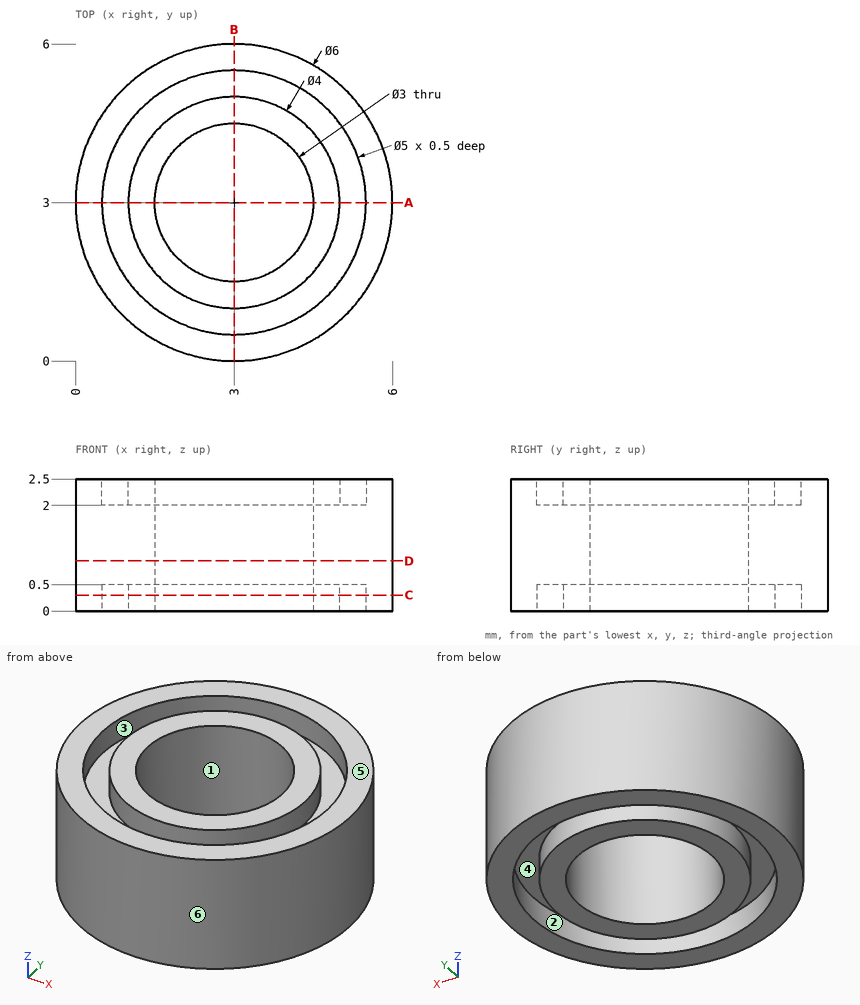
The figure shows three views and two pictorial views of one solid part (mm, origin at its lowest corner). Answer the questions. A direction names the side the tool comes from. Round coordinates to 2 decimals unless told otherwise and drop trailing zeros. Order: outer loops, then holes, each group sorted by start corner. A loop starts at its lowest first (then second) coordinate and runs counter-clockwise, first axis right, second up. Notation, with made-up numbers: M 33,40.25 L 61,40.25 A23 cw 61,61.25 Z; hole C -28.75,3 d1. An arc over 180 degrees is marked long. Answer in a Markdown table with one row per item. Add a question column.
1) The part is cut by section A-A on y = 3. Determine the outline of the cut face in (x, z), plus the area to 3 significant figures.
2) Which of the six approach directions +Z, -Z, +X, -X, +Y, -Y give full straight-line access (tool end or side, diameter ignored) to the marked faces 1, 2 and 3?
3) Determine the mould class of the marked faces 4, 5 and 6 for opening direction X: pulls with the +X half, pulls with the -X half, needs draft (parallel to the pull), parting line crosses it, or undercut.
4) The part is cut by section C-C on z = 0.3. Determine the outline of the cut face in (x, y).
5) A flat-ended cylindrical pin translates along its axis: pin 1 Ø1.5 at (y, z) = (5, 1.5) entering from +X. Find the tip coordinate at first contact, or state that the pin passes through.
6) Consider line 1 along Y through (x, z) = (3, 0.2); line 2 along Y through (x, z) = (3, 1.85); line 3 along Y through (x, z) = (1.9, 0.3) (3 decimals). Determine where each line is inside the solid, lowest interval first. Write a range as from..to.
7) The part is cut by section D-D on z = 0.95. Determine the outline of the cut face in (x, y).
Findings below:
| question | item | result |
|---|---|---|
| 1 | outline | M 0,0 L 0.5,0 L 0.5,0.5 L 1,0.5 L 1,0 L 1.5,0 L 1.5,2.5 L 1,2.5 L 1,2 L 0.5,2 L 0.5,2.5 L 0,2.5 Z; M 4.5,0 L 5,0 L 5,0.5 L 5.5,0.5 L 5.5,0 L 6,0 L 6,2.5 L 5.5,2.5 L 5.5,2 L 5,2 L 5,2.5 L 4.5,2.5 Z |
| 1 | area | 6.50 mm² |
| 2 | face 1 | +Z, -Z |
| 2 | face 2 | -Z |
| 2 | face 3 | +Z |
| 3 | face 4 | undercut |
| 3 | face 5 | needs draft |
| 3 | face 6 | parting line crosses it |
| 4 | outline | C 3,3 d6; C 3,3 d4; hole C 3,3 d5; hole C 3,3 d3 |
| 5 | pin 1 | stops at x = 5.73 |
| 6 | line 1 | y = 0..0.5, 1..1.5, 4.5..5, 5.5..6 |
| 6 | line 2 | y = 0..1.5, 4.5..6 |
| 6 | line 3 | y = 0.209..0.755, 1.33..1.98, 4.02..4.67, 5.245..5.791 |
| 7 | outline | C 3,3 d6; hole C 3,3 d3 |
